Design review of the part shown in the three views and the two pictorial views. Dimensions are in mm from the part's minimum x, y and z. A direction names the side the tool comes from. Give positions to 0.01 mm unless a question says otherwise; leave off trailing zeros. Write each loop counter-clockwise with the first axis right and the second up, starting at its lowest first coordinate (ties: lowest second). Pieces come first, ordered by that corner, then holes. Notation, with made-up numbers: (-39, 42.5) -> (-17, 42.5) arc R10 ccw to (-17, 53.5) -> close; hole circle Ø6 at (12, 46). An arc over 180 degrees is marked (long way). Use CSV: the item, a comma, the result in double quotes.
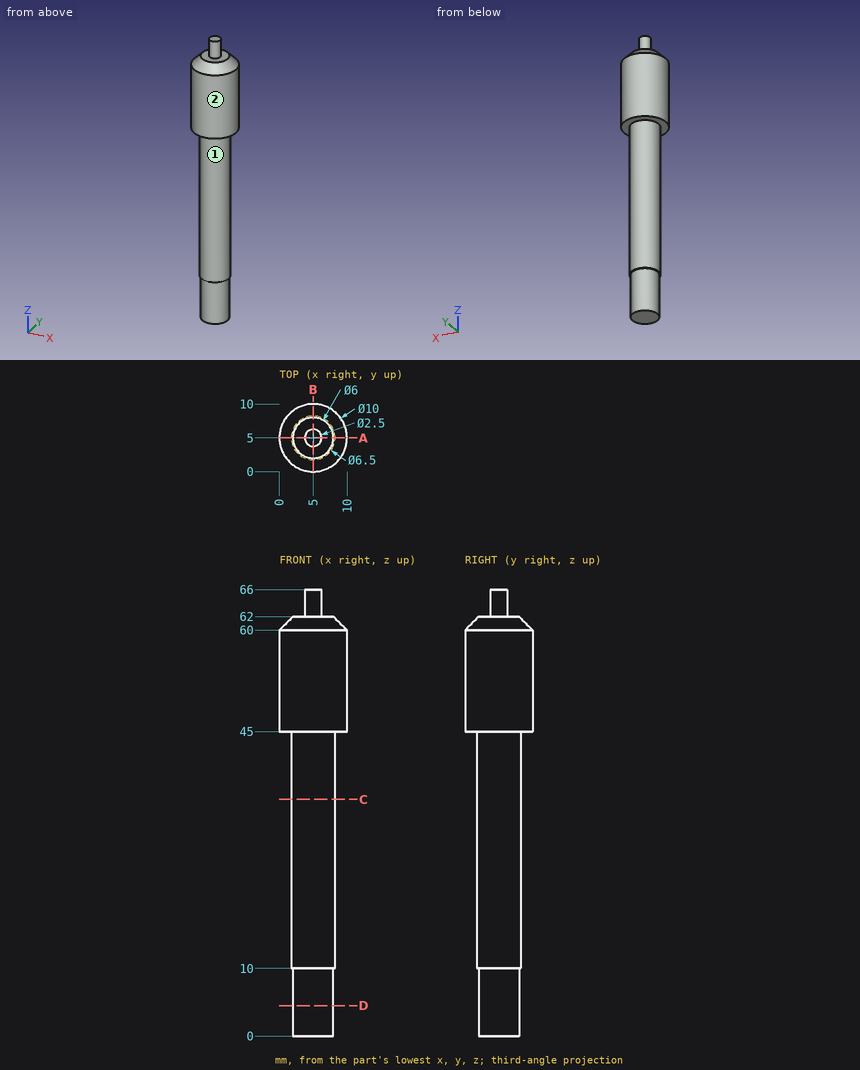
Q1. Consider section C-C (z = 35). Write out the cut boundary in (x, y).
Derived:
outline,"circle Ø6.5 at (5, 5)"
Q2. Consider section D-D (z = 4.5). Write out the cut boundary in (x, y).
Derived:
outline,"circle Ø6 at (5, 5)"
Q3. Consider section A-A (y = 5). Write out the cut boundary in (x, z), then the cut area to 4 significant figures.
Derived:
outline,"(0, 45) -> (1.75, 45) -> (1.75, 10) -> (2, 10) -> (2, 0) -> (8, 0) -> (8, 10) -> (8.25, 10) -> (8.25, 45) -> (10, 45) -> (10, 60) -> (8, 62) -> (6.25, 62) -> (6.25, 66) -> (3.75, 66) -> (3.75, 62) -> (2, 62) -> (0, 60) -> close"
area,"463.5 mm2"
Q4. Insertion check: pin 1 (3 mm diameter, centred on y = 8, z = 27.5, fed in from -X); pin 2 (1.5 mm diameter, centred on x = 6.5, z = 37, fed in from +Y); pin 3 (3 mm diameter, centred on x = 4.5, y = 8, fed in from +Z). Each pin has a flat end and moves straight along its axis. Give the tip position at first contact, or say it passes through.
Derived:
pin 1,"stops at x = 2.12"
pin 2,"stops at y = 8.16"
pin 3,"stops at z = 62"
Q5. To check wall thickness, follow probe 1 along Z at (x, y) = (2.5, 6); probe 2 along Y at (x, z) = (6.25, 18.5); probe 3 along Y at (x, z) = (3, 47). State the ranges of each line that lie inside material, in increasing order.
Derived:
probe 1,"z = 0 to 62"
probe 2,"y = 2 to 8"
probe 3,"y = 0.42 to 9.58"
Q6. Machinability: for the marked faces 1 and 2, which of the approach directions +Z, -Z, +X, -X, +Y, -Y give a long, thin tool a straight path to every point of the face, cutting with its end or side? Answer none if there is none.
Derived:
face 1,"-Z"
face 2,"+Z, -Z"
